from build123d import *

# Parameters (mm, degrees)
SKETCH1_W            = 20
SKETCH1_H            = 6.35
SKETCH1_W_2          = 6.35
SKETCH1_H_2          = 20
BOSS_EXTRUDE1_DEPTH  = 38.1
SKETCH2_W            = 26.11
SKETCH2_H            = 26.35
BOSS_EXTRUDE2_DEPTH  = 6.81899017
BOSS_EXTRUDE3_DEPTH  = 2.54
BOSS_EXTRUDE4_DEPTH  = 2.54
BOSS_EXTRUDE5_DEPTH  = 2.54
M4_CLEARANCE_HOLE1_D = 4.5
M4_CLEARANCE_HOLE2_D = 4.5


with BuildPart() as part:
    # Sketch1 → Boss-Extrude1 (new body)
    with BuildSketch(Plane(origin=(0, 0, 0), x_dir=(1, 0, 0), z_dir=(0, 1, 0))):
        with Locations((10, -3.175)):
            Rectangle(SKETCH1_W, SKETCH1_H)
        with Locations((-3.175, -3.175)):
            Rectangle(SKETCH1_W_2, SKETCH1_H)
        with Locations((-3.175, 10)):
            Rectangle(SKETCH1_W_2, SKETCH1_H_2)
    extrude(amount=BOSS_EXTRUDE1_DEPTH)

    # Sketch2 → Boss-Extrude2 (add)
    with BuildSketch(Plane(origin=(0, 38.1, 0), x_dir=(1, 0, 0), z_dir=(0, 1, 0))):
        with BuildLine():
            Line((-32.46, -58.81), (8.84, -58.81))
            Line((8.84, -58.81), (5.392081528, -55.362081528))
            ThreePointArc((5.392081528, -55.362081528), (3.539438165, -55.730595205), (2.49, -54.16))
            Line((2.49, -54.16), (-26.11, -54.16))
            ThreePointArc((-26.11, -54.16), (-27.159438165, -55.730595205), (-29.012081528, -55.362081528))
            Line((-29.012081528, -55.362081528), (-32.46, -58.81))
        make_face()
        with BuildLine():
            Line((5.392081528, -55.362081528), (8.84, -58.81))
            Line((8.84, -58.81), (8.84, -17.51))
            Line((8.84, -17.51), (5.392081528, -20.957918472))
            ThreePointArc((5.392081528, -20.957918472), (5.760595205, -21.509438165), (5.89, -22.16))
            ThreePointArc((5.89, -22.16), (5.392081528, -23.362081528), (4.19, -23.86))
            Line((4.19, -23.86), (4.19, -52.46))
            ThreePointArc((4.19, -52.46), (5.392081528, -52.957918472), (5.89, -54.16))
            ThreePointArc((5.89, -54.16), (5.760595205, -54.810561835), (5.392081528, -55.362081528))
        make_face()
        Polygon((20, -58.81), (20, -6.35), (-6.35, -6.35), (-32.46, -6.35), (-32.46, -17.51), (8.84, -17.51), (8.84, -58.81), align=None)
        with Locations((-19.405, 6.825)):
            Rectangle(SKETCH2_W, SKETCH2_H)
        with BuildLine():
            Line((8.84, -17.51), (-32.46, -17.51))
            Line((-32.46, -17.51), (-29.012081528, -20.957918472))
            ThreePointArc((-29.012081528, -20.957918472), (-27.159438165, -20.589404795), (-26.11, -22.16))
            Line((-26.11, -22.16), (2.49, -22.16))
            ThreePointArc((2.49, -22.16), (3.539438165, -20.589404795), (5.392081528, -20.957918472))
            Line((5.392081528, -20.957918472), (8.84, -17.51))
        make_face()
        with BuildLine():
            Line((-29.012081528, -20.957918472), (-32.46, -17.51))
            Line((-32.46, -17.51), (-32.46, -58.81))
            Line((-32.46, -58.81), (-29.012081528, -55.362081528))
            ThreePointArc((-29.012081528, -55.362081528), (-29.380595205, -53.509438165), (-27.81, -52.46))
            Line((-27.81, -52.46), (-27.81, -23.86))
            ThreePointArc((-27.81, -23.86), (-29.380595205, -22.810561835), (-29.012081528, -20.957918472))
        make_face()
        with BuildLine():
            ThreePointArc((-26.607918472, -23.362081528), (-27.159438165, -23.730595205), (-27.81, -23.86))
            Line((-27.81, -23.86), (-27.81, -52.46))
            ThreePointArc((-27.81, -52.46), (-27.159438165, -52.589404795), (-26.607918472, -52.957918472))
            Line((-26.607918472, -52.957918472), (-22.7220672, -49.0720672))
            ThreePointArc((-22.7220672, -49.0720672), (-27.241993428, -38.16), (-22.7220672, -27.2479328))
            Line((-22.7220672, -27.2479328), (-26.607918472, -23.362081528))
        make_face()
        with BuildLine():
            Line((2.49, -22.16), (-26.11, -22.16))
            ThreePointArc((-26.11, -22.16), (-26.239404795, -22.810561835), (-26.607918472, -23.362081528))
            Line((-26.607918472, -23.362081528), (-22.7220672, -27.2479328))
            ThreePointArc((-22.7220672, -27.2479328), (-11.81, -22.728006572), (-0.8979328, -27.2479328))
            Line((-0.8979328, -27.2479328), (2.987918472, -23.362081528))
            ThreePointArc((2.987918472, -23.362081528), (2.619404795, -22.810561835), (2.49, -22.16))
        make_face()
        with BuildLine():
            Line((-0.8979328, -49.0720672), (2.987918472, -52.957918472))
            ThreePointArc((2.987918472, -52.957918472), (3.539438165, -52.589404795), (4.19, -52.46))
            Line((4.19, -52.46), (4.19, -23.86))
            ThreePointArc((4.19, -23.86), (3.539438165, -23.730595205), (2.987918472, -23.362081528))
            Line((2.987918472, -23.362081528), (-0.8979328, -27.2479328))
            ThreePointArc((-0.8979328, -27.2479328), (2.447302874, -32.254431787), (3.621993428, -38.16))
            ThreePointArc((3.621993428, -38.16), (2.447302874, -44.065568213), (-0.8979328, -49.0720672))
        make_face()
        with BuildLine():
            Line((-26.11, -54.16), (2.49, -54.16))
            ThreePointArc((2.49, -54.16), (2.619404795, -53.509438165), (2.987918472, -52.957918472))
            Line((2.987918472, -52.957918472), (-0.8979328, -49.0720672))
            ThreePointArc((-0.8979328, -49.0720672), (-11.81, -53.591993428), (-22.7220672, -49.0720672))
            Line((-22.7220672, -49.0720672), (-26.607918472, -52.957918472))
            ThreePointArc((-26.607918472, -52.957918472), (-26.239404795, -53.509438165), (-26.11, -54.16))
        make_face()
    extrude(amount=-BOSS_EXTRUDE2_DEPTH)

    # Sketch3 → Boss-Extrude3 (add)
    with BuildSketch(Plane(origin=(20, 0, 0), x_dir=(0, 0, -1), z_dir=(1, 0, 0))):
        Polygon((-58.81, 31.28100983), (-6.35, 0), (-6.35, 31.28100983), align=None)
    extrude(amount=-BOSS_EXTRUDE3_DEPTH)

    # Sketch4 → Boss-Extrude4 (add)
    with BuildSketch(Plane(origin=(0, 0, -20), x_dir=(-1, 0, 0), z_dir=(0, 0, -1))):
        Polygon((6.35, 0), (32.46, 31.28100983), (6.35, 31.28100983), align=None)
    extrude(amount=-BOSS_EXTRUDE4_DEPTH)

    # Sketch5 → Boss-Extrude5 (add)
    with BuildSketch(Plane.XY.offset(6.35)):
        Polygon((-6.35, -0.46899017), (-32.46, 31.28100983), (-6.35, 31.28100983), align=None)
    extrude(amount=-BOSS_EXTRUDE5_DEPTH)

    # M4 Clearance Hole1 (through all)
    with Locations(Plane.ZY.offset(6.35)):
        with Locations((-10, 23.460757372), (-10, 7.820252457)):
            Hole(M4_CLEARANCE_HOLE1_D / 2)

    # M4 Clearance Hole2 (through all)
    with Locations(Plane.XY.offset(6.35)):
        with Locations((10, 7.820252457), (10, 23.460757372)):
            Hole(M4_CLEARANCE_HOLE2_D / 2)


solid = part.part
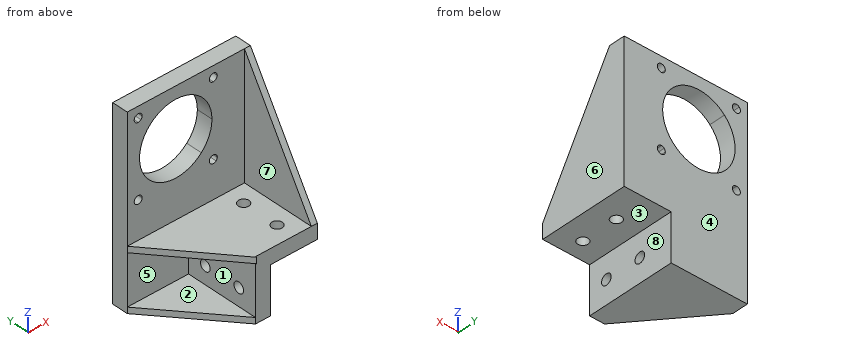
The model under review builds one solid part; all positions refer to its coordinate system, in mm. Face numbers are marked on the shaded views. A direction names the side the tool comes from. Give positions to 0.01 mm unless a question says otherwise; leave off trailing zeros. Loops run counter-clockwise (first coordinate to the right, second up) from the corner with the lowest first, then second, coordinate; pieces in that order, holes last. Notation, with made-up numbers: (32.5, -33.75) -> (42.5, -33.75) arc R23 ccw to (42.5, -16.75) -> close; hole circle Ø5 at (-29.5, -2). An arc over 180 degrees is marked (long way). Write each question's results on one line, items separated by ' | '.
1) Draft analysis for pull direction Z (two halves, no side actions). For the marked faces 1, 2, 3 and 4, state which applies: pulls with the +Z half, pulls with the -Z half, needs draft (parallel to the pull), parting line crosses it, or undercut.
Conclusion:
face 1: undercut | face 2: undercut | face 3: pulls with the -Z half | face 4: needs draft
2) Tool access review of the marked faces 5, 6, 7 and 8: name each direction out of +Z, -Z, +X, -X, +Y, -Y from which nothing blocks a thin tool from reaching the whole face with its end or side.
Conclusion:
face 5: -X, -Y | face 6: +Z, -Z, +X, +Y, -Y | face 7: +Z, -X, -Y | face 8: -Z, +X, +Y, -Y
3) Take a section at D-D, the plane z = 7.5. Give the boundary of the cut face in (x, y), plus the area to 3 significant figures.
Conclusion:
outline: (-32.46, 31.28) -> (17.46, 31.28) -> (17.46, 0.69) -> (20, 0.69) -> (20, 38.1) -> (-32.46, 38.1) -> close | area: 435 mm^2
4) Take a section at B-B, the plane x = 10. Give the boundary of the cut face in (y, z).
Conclusion:
outline: (0, 0) -> (5.57, 0) -> (5.57, 6.35) -> (0, 6.35) -> close; (10.07, 0) -> (21.21, 0) -> (21.21, 6.35) -> (10.07, 6.35) -> close; (25.71, 0) -> (38.1, 0) -> (38.1, 58.81) -> (31.28, 58.81) -> (31.28, 6.35) -> (25.71, 6.35) -> close
5) Take a section at C-C, the plane x = -18. Give the boundary of the cut face in (y, z), plus the area to 3 significant figures.
Conclusion:
outline: (13.7, 3.81) -> (31.28, 3.81) -> (31.28, -17.46) -> (13.96, -17.46) -> (13.96, -20) -> (38.1, -20) -> (38.1, 24.02) -> (31.28, 24.02) -> (31.28, 6.35) -> (13.7, 6.35) -> close; (31.28, 52.3) -> (38.1, 52.3) -> (38.1, 58.81) -> (31.28, 58.81) -> close | area: 433 mm^2
6) For line 1 along Y through (x, z) = (-1, -10); line 2 along Z through (x, y) = (-21, 21); line 3 along Z through (x, y) = (-12, 36), list the stretches that pass through material, from the lowest coordinate up. Write a range as from..to.
Conclusion:
line 1: y = 0..5.57, 10.07..21.21, 25.71..38.1 | line 2: z = -20..-17.46, 3.81..6.35 | line 3: z = -20..22.73, 53.59..58.81
7) Insertion check: pin 1 Ø10 at (x, y) = (10, 16.5) entering from -Z; pin 2 Ø12 at (x, y) = (3.5, 16.5) entering from +Z; pin 3 Ø12 at (y, z) = (10, 37) entering from -X; pin 4 Ø6.5 at (y, z) = (18, -6.5) entering from -X. Each pin has a flat end and moves straight along its axis. Give the tip position at first contact, or say it passes through.
Conclusion:
pin 1: stops at z = 0 | pin 2: stops at z = 6.35 | pin 3: passes through | pin 4: stops at x = -6.35
8) Take a section at A-A, the plane z = -10. Give the boundary of the cut face in (x, y), plus the area to 3 significant figures.
Conclusion:
outline: (-32.46, 31.28) -> (-6.35, 31.28) -> (-6.35, 25.71) -> (0, 25.71) -> (0, 38.1) -> (-32.46, 38.1) -> close; (-6.35, 0) -> (0, 0) -> (0, 5.57) -> (-6.35, 5.57) -> close; (-6.35, 10.07) -> (0, 10.07) -> (0, 21.21) -> (-6.35, 21.21) -> close | area: 363 mm^2
